from build123d import *

# Parameters (mm, degrees)
F1_DEPTH        = 2.54
F2_DEPTH        = 2.54
F2_COPIES_COUNT = 5
F2_COPIES_ANGLE = 105
F3_R            = 2.159
F4_DEPTH        = 12.7


# Not quite as in the source:
# - a pattern or mirror of a feature is missing from the dataset's text; its kind, count and spacing are read off the source's solid


with BuildPart() as f1:
    # F0 (on Front) → F1 (new body)
    with BuildSketch(Plane.XZ):
        with BuildLine():
            ThreePointArc((-1.6725612742, 11.9485046673), (-7.917852399, -9.1033970795), (12.065, 0))
            ThreePointArc((12.065, 0), (9.1033970795, 7.917852399), (1.6725612742, 11.9485046673))
            ThreePointArc((1.6725612742, 11.9485046673), (0, 12.065), (-1.6725612742, 11.9485046673))
        make_face()
    extrude(amount=F1_DEPTH)

    # F0 (on Front) → F2 (join, through all)
    with BuildSketch(Plane.XZ):
        with BuildLine():
            ThreePointArc((-1.6725612742, 11.9485046673), (0, 12.065), (1.6725612742, 11.9485046673))
            add(Edge.make_bspline(
                [(1.6725612742, 11.9485046673), (1.6184790505, 12.4941120183), (1.4671756256, 13.4121286243), (0.8625889567, 14.3194638744), (0.635, 14.478)],
                knots=[0, 0, 0, 0, 0.5287892811, 1, 1, 1, 1], degree=3))
            Line((0.635, 14.478), (-0.635, 14.478))
            add(Edge.make_bspline(
                [(-1.6725612742, 11.9485046673), (-1.6184790505, 12.4941120183), (-1.4671756256, 13.4121286243), (-0.8625889567, 14.3194638744), (-0.635, 14.478)],
                knots=[0, 0, 0, 0, 0.5287892811, 1, 1, 1, 1], degree=3))
        make_face()
    f2 = extrude(amount=F2_DEPTH)

    # F2_copies: F2 ×5 about axis
    f2_copies_axis = Axis((0, 0, 0), (0, 1, 0))
    for i in range(1, F2_COPIES_COUNT):
        add(f2.rotate(f2_copies_axis, i * F2_COPIES_ANGLE / (F2_COPIES_COUNT - 1)))

    # F3 (on face) → F4 (join)
    with BuildSketch(Plane.XZ.offset(2.54)):
        Circle(F3_R)
    extrude(amount=F4_DEPTH)


solid = f1.part
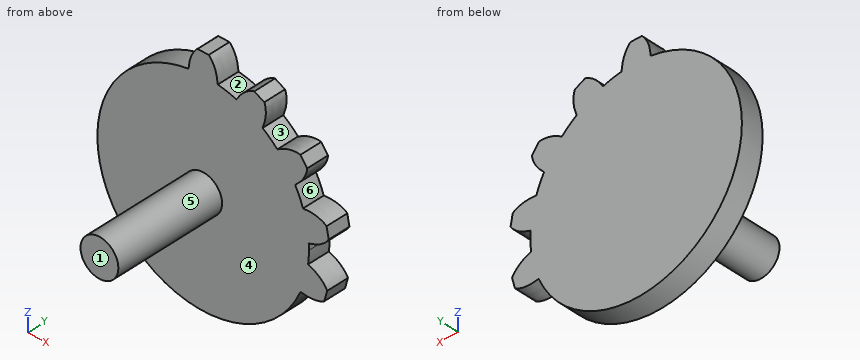
Part model, mm, in its own coordinate system. Face numbers are marked on the shaded views. A direction names the side the tool comes from. Coordinates: 2 decimals unless noted, no trailing zeros. Loops run counter-clockwise (first coordinate to the right, second up) from the corner with the lowest first, then second, coordinate; pieces in that order, holes last. Notation, with made-up numbers: (-18, -6.75) - (3, -6.75) arc R22 ccw to (3, 22.25) - close; hole circle Ø4 at (-20.75, -22.5). An arc over 180 degrees is marked (long way). Write each question's results on one line, items separated by ' | '. Start each with the question number.
Q1. Slice it at A-A on x = 0. Give the cut face in (y, z) (3 decimals).
Q2. Slice it at B-B on y = -10. Give the cut face in (x, z), and give its area (3 significant figures).
Q3. Drop flat-ended pins along their axis: pin 1 Ø3 at (x, z) = (9, 9.5) entering from -Y; pin 2 Ø2 at (y, z) = (-8.5, -1.5) entering from +X; pin 3 Ø3 at (y, z) = (-5, 8) entering from +X; pin 4 Ø4 at (y, z) = (-6.5, 1.5) entering from -X. Give the stop position or say it passes through.
Q4. Which spindle directions (+Z, -Z, +X, -X, +Y, -Y) get a long thin tool onto all of the face, cutting with end or side? Do the marked faces 1, 2 and 3. Say none if no direction does.
Q5. Two-plate mould, pull along Z, no slides. Class the marked faces 4, 5 and 6: +Z half, -Z half, draft (parallel to the pull), parting line (faces both ways), or undercut.
Q6. Slice it at D-D on x = -6.5. Give the cut face in (y, z), and give its area (3 significant figures).
Q7. Probe line 1 along Y through (x, z) = (8.25, -6.25); line 2 along Z through (x, y) = (1.25, -7); line 3 along Z through (x, y) = (-10.5, -1.75). List the from-to ranges inside material, lowest first.
Q8. Slice it at C-C on z = 4.75. Give the cut face in (x, y).
Answer:
1) outline: (-15.24, -2.159) - (-2.54, -2.159) - (-2.54, -12.065) - (0, -12.065) - (0, 14.478) - (-2.54, 14.478) - (-2.54, 2.159) - (-15.24, 2.159) - close
2) outline: circle Ø4.32 at (0, 0) | area: 14.6 mm2
3) pin 1: stops at y = -2.54 | pin 2: stops at x = 2.1 | pin 3: passes through | pin 4: stops at x = -2.16
4) face 1: +Z, -Z, +X, -X, -Y | face 2: +Z, +Y, -Y | face 3: +Y, -Y
5) face 4: draft | face 5: parting line | face 6: undercut
6) outline: (-2.54, -10.16) - (0, -10.16) - (0, 10.16) - (-2.54, 10.16) - close | area: 51.6 mm2
7) line 1: y = -2.54 to 0 | line 2: z = -1.76 to 1.76 | line 3: z = -5.94 to 5.94
8) outline: (-11.09, -2.54) - (11.09, -2.54) - (11.09, 0) - (-11.09, 0) - close
